Verification items for the finished model (mm, model axes). A direction names the side the tool comes from. Coordinates: 2 decimals unless noted, no trailing zeros. Order: outer loops, then holes, each group sorted by start corner. A loop starts at its lowest first (then second) coordinate and runs counter-clockwise, first axis right, second up. Notation, with made-up numbers: (-4, 68.25) - (4, 68.25) arc R28 cw to (4, 89.25) - close; hole circle Ø1 at (60, 54). An arc over 180 degrees is marked (long way). One line per question, with ' | ' between items. Start each with the question number.
from build123d import *

# Parameters (mm, degrees)
F0_R     = 20.44695
F0_R_2   = 10.086929
F0_R_3   = 5.276256
F1_DEPTH = 25.4
F2_DEPTH = 50.8


with BuildPart() as f1:
    # F0 (on Front) → F1 (new body)
    with BuildSketch(Plane.XZ):
        Circle(F0_R)
        Circle(F0_R_2, mode=Mode.SUBTRACT)
        Circle(F0_R_2)
        Circle(F0_R_3, mode=Mode.SUBTRACT)
        Circle(F0_R_3)
    extrude(amount=F1_DEPTH)

    # F0 (on Front) → F2 (join)
    with BuildSketch(Plane.XZ):
        Circle(F0_R_2)
        Circle(F0_R_3, mode=Mode.SUBTRACT)
    extrude(amount=F2_DEPTH)


solid = f1.part
Item 1: Section check C-C (y = -46). Record the cut outline in (x, z).
Item 2: Thickness scan on probe 1 along Z at (x, y) = (0, -45.5); probe 2 along Y at (x, z) = (13.5, -6.5). Record the ranges inside material, lowest first. Write a range as from..to.
Item 3: Section check A-A (z = 0). Record the cut outline in (x, y).
Item 4: Section check D-D (y = -10.5). Record the cut outline in (x, z), then the cut area to 3 significant figures.
Item 5: Mould release check, pull along X, two halves, no side actions. Record for faces 3 (the flat face through (-9.4, -25.4, -4.3)), 4 (the flat face through (0, -25.4, 0)), 5 (the cylindrical face through (-8.005, -37.922, -6.138)): +X half, -X half, draft (parallel to the pull), parting line (faces both ways), or undercut.
Item 6: Section check B-B (x = 0). Record the cut outline in (y, z), then the cut area to 3 significant figures.
Item 7: Set-up check for faces 1 (the cylindrical face through (-16.226, -12.522, -12.442)), 2 (the cylindrical face through (-1.14, -37.92, -5.15)): record each of +Z, -Z, +X, -X, +Y, -Y from which the full face is reachable in a straight line by a thin tool's end or side.
Item 8: Gauge pin test, flat ends, axial feed: pin 1 (10 mm diameter, centred on y = -7, z = -12, fed in from -X); pin 2 (4 mm diameter, centred on x = 11.5, z = 12.5, fed in from -Y); pin 3 (1.5 mm diameter, centred on y = -40.5, z = -4.5, fed in from -X). Record the tip position at first contact, or that the pin passes through.
Completed:
1) outline: circle Ø20.17 at (0, 0); hole circle Ø10.55 at (0, 0)
2) probe 1: z = -10.09..-5.28, 5.28..10.09 | probe 2: y = -25.4..0
3) outline: (-20.45, -25.4) - (-10.09, -25.4) - (-10.09, -50.8) - (-5.28, -50.8) - (-5.28, -25.4) - (5.28, -25.4) - (5.28, -50.8) - (10.09, -50.8) - (10.09, -25.4) - (20.45, -25.4) - (20.45, 0) - (-20.45, 0) - close
4) outline: circle Ø40.89 at (0, 0) | area: 1,310 mm^2
5) face 3: draft | face 4: undercut | face 5: parting line
6) outline: (-50.8, -10.09) - (-25.4, -10.09) - (-25.4, -20.45) - (0, -20.45) - (0, 20.45) - (-25.4, 20.45) - (-25.4, 10.09) - (-50.8, 10.09) - (-50.8, 5.28) - (-25.4, 5.28) - (-25.4, -5.28) - (-50.8, -5.28) - close | area: 1,280 mm^2
7) face 1: +Y, -Y | face 2: -Y
8) pin 1: stops at x = -19.21 | pin 2: stops at y = -25.4 | pin 3: stops at x = -9.36
